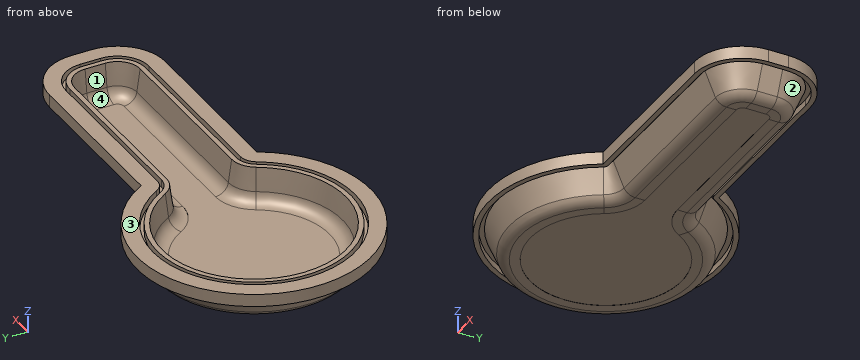
```python
from build123d import *

# Parameters (mm, degrees)
F3_DEPTH = 1.5


with BuildPart() as f2:
    # F2: sweep along a path in F1
    with BuildLine(Plane.XY) as f2_path:
        ThreePointArc((107.5000001721, -6.5), (109.267767163, -5.7677669149), (110.0000001721, -3.9999998925))
        Line((110.0000001721, -3.9999998925), (109.9999998279, 4.0000001075))
        ThreePointArc((109.9999998279, 4.0000001075), (109.2677667429, 5.767766991), (107.4999998279, 6.5))
        Line((107.4999998279, 6.5), (40.4134878475, 6.5))
        ThreePointArc((40.4134878475, 6.5), (32.1192516055, 8.7362121033), (26.0732179661, 14.8387096774))
        ThreePointArc((26.0732179661, 14.8387096774), (-30, 0), (26.0732179661, -14.8387096774))
        ThreePointArc((26.0732179661, -14.8387096774), (32.1192516055, -8.7362121033), (40.4134878475, -6.5))
        Line((40.4134878475, -6.5), (107.5000001721, -6.5))
    # F0 (on Front) → F2 (sweep)
    with BuildSketch(Plane.XZ):
        with BuildLine():
            Line((-33.8218298437, -0.093526227), (-30, -0.0597173114))
            Line((-30, -0.0597173114), (-30, 1.4402826886))
            ThreePointArc((-30, 1.4402826886), (-33.4331031287, 2.5807074242), (-35.1984127671, 5.7383089745))
            Line((-35.1984127671, 5.7383089745), (-36.5, 14.9995833623))
            Line((-36.5, 14.9995833623), (-38.45, 14.9995833623))
            Line((-38.45, 14.9995833623), (-38.45, 11.9995833623))
            Line((-38.45, 11.9995833623), (-40.05, 11.9995833623))
            Line((-40.05, 11.9995833623), (-40.05, 15))
            Line((-40.05, 15), (-46.5, 15))
            Line((-46.5, 15), (-46.5, 10))
            Line((-46.5, 10), (-44.5, 10))
            Line((-44.5, 10), (-44.5, 12.5))
            Line((-44.5, 12.5), (-42.5, 12.5))
            Line((-42.5, 12.5), (-38.2571726182, 2.515018017))
            ThreePointArc((-38.2571726182, 2.515018017), (-36.400812876, 0.5964028574), (-33.8218298437, -0.093526227))
        make_face()
    sweep(path=f2_path.line)

    # F1 (on Top) → F3 (join)
    with BuildSketch(Plane.XY):
        with BuildLine():
            Line((40.4134878475, -6.5), (107.5000001721, -6.5))
            ThreePointArc((107.5000001721, -6.5), (109.267767163, -5.7677669149), (110.0000001721, -3.9999998925))
            Line((110.0000001721, -3.9999998925), (109.9999998279, 4.0000001075))
            ThreePointArc((109.9999998279, 4.0000001075), (109.2677667429, 5.767766991), (107.4999998279, 6.5))
            Line((107.4999998279, 6.5), (40.4134878475, 6.5))
            ThreePointArc((40.4134878475, 6.5), (32.1192516055, 8.7362121033), (26.0732179661, 14.8387096774))
            ThreePointArc((26.0732179661, 14.8387096774), (-30, 0), (26.0732179661, -14.8387096774))
            ThreePointArc((26.0732179661, -14.8387096774), (32.1192516055, -8.7362121033), (40.4134878475, -6.5))
        make_face()
    extrude(amount=F3_DEPTH)


solid = f2.part
```
Could you check a few things on this model? Use its own coordinates, in mm. Face numbers are marked on the shaded views. A direction names the side the tool comes from. Give positions to 0.01 mm unless a question says otherwise; leave off trailing zeros. Write each question's results on one line, items separated by ' | '.
1. I need wall thicknesses on L1, parallel to Y at x = 0, z = 11.9; L2, parallel to Y at x = 61, z = 12.75; L3, parallel to Z at x = -25, y = 12. Which ranges of each line are inside material? Lowest first, please.
Check sheet entries:
L1: y = -46.5 to -44.5, -42.25 to -36.06, 36.06 to 42.25, 44.5 to 46.5 | L2: y = -23 to -16.55, -14.95 to -12.68, 12.68 to 14.95, 16.55 to 23 | L3: z = 0 to 1.5
2. On a 3-axis mill with a long thin cutter (end or side, diameter ignored), from which of +Z, -Z, +X, -X, +Y, -Y can I reach the whole of each face in a straight line? I mean the marked faces 1 and 2. Say none if no direction works.
Check sheet entries:
face 1: +Z | face 2: -Z
3. Will these pins go through, and if not, where does the flat tip stop? pin 1 Ø2.5 at (x, z) = (76.5, 12.5) entering from -Y; pin 2 Ø6 at (x, z) = (20, 4.5) entering from -Y; pin 3 Ø18 at (x, y) = (11, -6.5) entering from +Z.
Check sheet entries:
pin 1: stops at y = -23 | pin 2: stops at y = -35.78 | pin 3: stops at z = 1.5
4. If we mould it in two halves opening along X, with no side actions, what happens to the marked faces 3 and 4? For each: released by +X, released by -X, zero draft, split by the parting line, or undercut.
Check sheet entries:
face 3: zero draft | face 4: undercut
